from build123d import *

# Parameters (mm, degrees)
F0_R      = 20.2700767199
F0_R_2    = 19.1
F1_DEPTH  = 25
F0_R_3    = 2
F2_DEPTH  = 2
F4_DEPTH  = 5
F3_W      = 13
F3_H      = 13
F3_R      = 2
F5_DEPTH  = 10
F7_DEPTH  = 13
F8_R      = 19
F9_DEPTH  = 25
F10_R     = 2.5
F11_DEPTH = 5
F12_SIZE  = 1


with BuildPart() as f1:
    # F0 (on Top) → F1 (new body)
    with BuildSketch(Plane.XY):
        Circle(F0_R)
        Circle(F0_R_2, mode=Mode.SUBTRACT)
    extrude(amount=-F1_DEPTH)

    # F0 (on Top) → F2 (join)
    with BuildSketch(Plane.XY):
        Circle(F0_R)
        Circle(F0_R_2, mode=Mode.SUBTRACT)
        Circle(F0_R_2)
        Circle(F0_R_3, mode=Mode.SUBTRACT)
    extrude(amount=F2_DEPTH)

    # F0 (on Top) → F4 (cut)
    with BuildSketch(Plane.XY):
        Circle(F0_R_3)
    extrude(amount=F4_DEPTH, mode=Mode.SUBTRACT)

    # F3 (on face) → F5 (join)
    with BuildSketch(Plane.XY):
        Rectangle(F3_W, F3_H)
        Circle(F3_R, mode=Mode.SUBTRACT)
    extrude(amount=F5_DEPTH)

    # F6 (on face) → F7 (join)
    with BuildSketch(Plane.XZ.offset(6.5)):
        with BuildLine():
            Line((-6.5, 13), (-6.5, 10))
            Line((-6.5, 10), (6.5, 10))
            Line((6.5, 10), (38.9184806049, 10))
            ThreePointArc((38.9184806049, 10), (41.4550102858, 10.2160216052), (43.9184806049, 10.8578643763))
            ThreePointArc((43.9184806049, 10.8578643763), (51.1659293188, 16.3397459622), (53.9184806049, 25))
            Line((53.9184806049, 25), (53.9184806049, 55.3070029616))
            Line((53.9184806049, 55.3070029616), (50.9184806049, 55.3070029616))
            Line((50.9184806049, 55.3070029616), (50.9184806049, 28))
            ThreePointArc((50.9184806049, 28), (46.5250823227, 17.3933982822), (35.9184806049, 13))
            Line((35.9184806049, 13), (-6.5, 13))
        make_face()
    extrude(amount=-F7_DEPTH)

    # F8 (on face) → F9 (join)
    with BuildSketch(Plane(origin=(50.9184806049, 0, 0), x_dir=(0, -1, 0), z_dir=(-1, 0, 0))):
        with Locations((0, 48.4660230577)):
            Circle(F8_R)
        with BuildLine():
            Line((-6.5, 55.3070029616), (-6.5, 30.6124519863))
            ThreePointArc((-6.5, 30.6124519863), (0, 29.4660230577), (6.5, 30.6124519863))
            Line((6.5, 30.6124519863), (6.5, 55.3070029616))
            Line((6.5, 55.3070029616), (-6.5, 55.3070029616))
        make_face()
    extrude(amount=F9_DEPTH)

    # F10 (on face) → F11 (join)
    with BuildSketch(Plane(origin=(25.9184806049, 0, 0), x_dir=(0, -1, 0), z_dir=(-1, 0, 0))):
        with Locations((0, 48.4660230577)):
            Circle(F10_R)
    extrude(amount=F11_DEPTH)

    # F12
    f12_edges = [f1.edges().sort_by_distance(p)[0] for p in [
        (20.918481, 2.5, 48.466023),
    ]]
    chamfer(f12_edges, length=F12_SIZE)


solid = f1.part
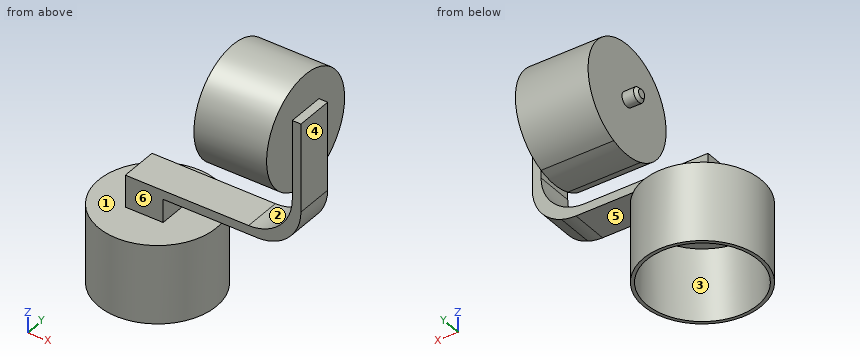
Geometry check sheet. Reference: the model listing, model coordinates, mm. Face numbers are marked on the shaded views. A direction names the side the tool comes from. Give positions to 0.01 mm unless a question says otherwise; leave off trailing zeros. Write each loop counter-clockwise with the first axis right and the second up, starting at its lowest first coordinate (ties: lowest second). Pieces come first, ordered by that corner, then holes. Notation, with made-up numbers: M -34,45 L -3,45 A27 ccw -3,79 Z; hole C -20.75,70.25 d11. An arc over 180 degrees is marked long. Answer as CSV lines item,"result". Start each with the question number.
Q1. Material ranges on L1, parallel to Y at x = 0, z = 6; L2, parallel to Y at x = 0, z = -14.75; L3, parallel to Z at x = 11, y = -5.5, recorded low to high.
Q2. Go/stop test with flat-tipped pins: pin 1 (3.5 mm diameter, centred on x = 0, y = 0, fed in from +Z); pin 2 (16 mm diameter, centred on x = 13, z = 19.5, fed in from -Y); pin 3 (6.5 mm diameter, centred on x = 18.5, y = -0.5, fed in from +Z). Record where each tip stops, or that it passes through.
Q3. Section check B-B, the plane x = 32.5. Record the cut outline in (y, z), then the cut area to 3 significant figures.
Q4. Section check D-D, the plane x = 0. Record the cut outline in (y, z), then the cut area to 3 significant figures.
Q5. Release check for a two-part mould opening along Z. For the marked faces 5 and 6 record: pulls with the +Z half, pulls with the -Z half, needs draft (parallel to the pull), parting line crosses it, or undercut.
Q6. Section check C-C, the plane y = -14. Record the cut outline in (x, z), then the cut area to 3 significant figures.
Q7. Tool access check on the marked faces 1, 2, 3 and 4. Record the directions out of +Z, -Z, +X, -X, +Y, -Y that give a thin tool (end or side, any length) a straight path to the whole face; none if there is none.
Geometry says:
1,L1,"-6.5 to -2, 2 to 6.5"
1,L2,"-20.27 to -19.1, 19.1 to 20.27"
1,L3,"0 to 2, 10 to 13"
2,pin 1,"z = 13"
2,pin 2,"y = -6.5"
2,pin 3,"z = 50.78"
3,outline,"C 0,48.47 d38; M -6.5,10 L 6.5,10 L 6.5,13 L -6.5,13 Z"
3,area,"1,170 mm^2"
4,outline,"M -20.27,-25 L -19.1,-25 L -19.1,0 L -2,0 L -2,10 L 2,10 L 2,0 L 19.1,0 L 19.1,-25 L 20.27,-25 L 20.27,2 L 6.5,2 L 6.5,13 L -6.5,13 L -6.5,2 L -20.27,2 Z"
4,area,"243 mm^2"
5,face 5,"undercut"
5,face 6,"needs draft"
6,outline,"M -14.66,-25 L -12.99,-25 L -12.99,0 L 12.99,0 L 12.99,-25 L 14.66,-25 L 14.66,2 L -14.66,2 Z; M 25.92,35.62 L 50.92,35.62 L 50.92,61.31 L 25.92,61.31 Z"
6,area,"784 mm^2"
7,face 1,"none"
7,face 2,"-X, +Y, -Y"
7,face 3,"-Z"
7,face 4,"+Z, -Z, +X, +Y, -Y"
